For this review, use the dimensioned drawing (mm, ordinates from the lowest corner) and the shaded views. A direction names the side the tool comes from. Coordinates: 2 decimals unless noted, no trailing zeros. Loops run counter-clockwise (first coordinate to the right, second up) from the corner with the lowest first, then second, coordinate; pieces in that order, holes last. Notation, with made-up numbers: M -11,20.5 L 47,20.5 A14 cw 47,28.5 Z; hole C 29.5,78 d11. An arc over 180 degrees is marked long. One line per item, written item: value.
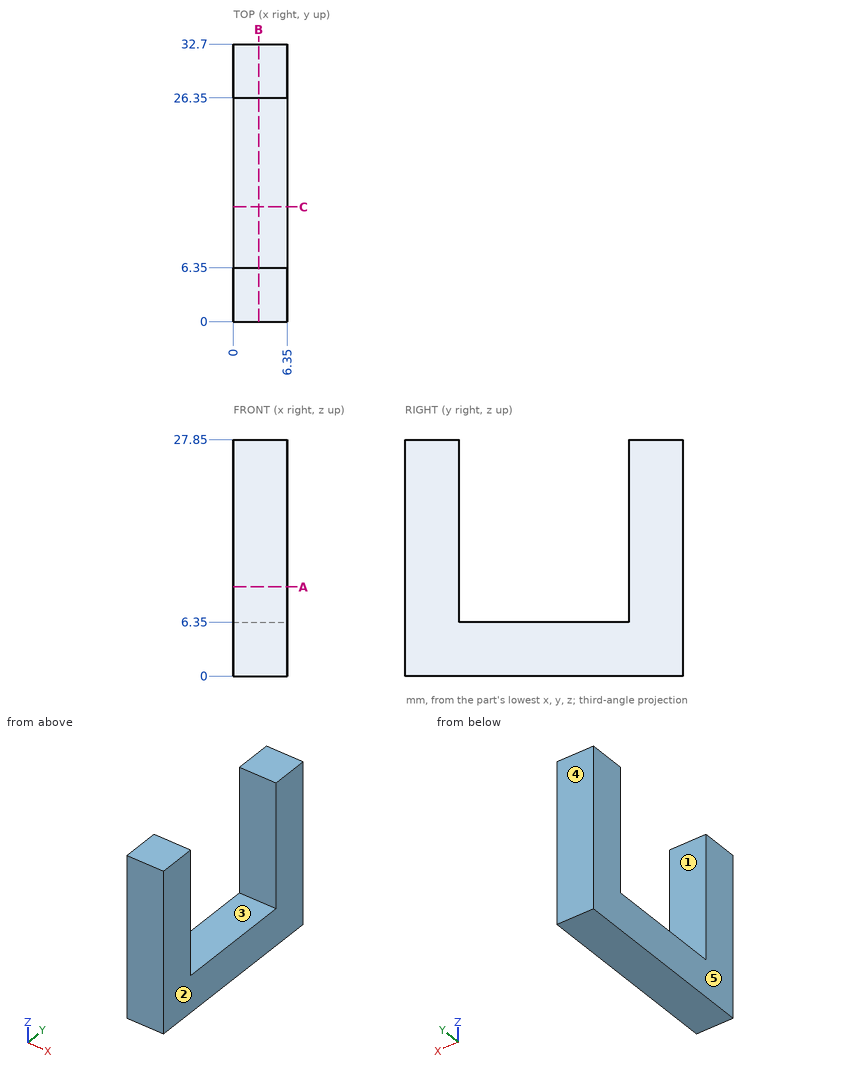
(1) We need section A-A on z = 10.5. State the section outline as (x, y) points, then the cut area to 3 significant figures.
Reply:
outline: M 0,0 L 6.35,0 L 6.35,6.35 L 0,6.35 Z; M 0,26.35 L 6.35,26.35 L 6.35,32.7 L 0,32.7 Z
area: 80.6 mm2
(2) Mouldability with a two-part tool opening along Y and no side actions: class the marked faces 3, 4 and 5 as released by +Y, released by -Y, zero draft, split by the parting line, or undercut.
Reply:
face 3: undercut
face 4: released by +Y
face 5: zero draft
(3) Tool access review of the marked faces 1 and 2: name each direction out of +Z, -Z, +X, -X, +Y, -Y from which nothing blocks a thin tool from reaching the whole face with its end or side.
Reply:
face 1: +Z, +X, -X
face 2: +Z, -Z, +X, +Y, -Y
(4) We need section C-C on y = 13.5. State the section outline as (x, z) points.
Reply:
outline: M 0,0 L 6.35,0 L 6.35,6.35 L 0,6.35 Z
(5) Insertion check: pin 1 (10 mm diameter, centred on y = 20, z = 10.5, fed in from +X); pin 2 (1.5 mm diameter, centred on x = 3.5, y = 23, fed in from +Z). Each pin has a flat end and moves straight along its axis. Give the tip position at first contact, or say it passes through.
Reply:
pin 1: stops at x = 6.35
pin 2: stops at z = 6.35
(6) We need section B-B on x = 3. State the section outline as (y, z) points, then the cut area to 3 significant figures.
Reply:
outline: M 0,0 L 32.7,0 L 32.7,27.85 L 26.35,27.85 L 26.35,6.35 L 6.35,6.35 L 6.35,27.85 L 0,27.85 Z
area: 481 mm2
(7) To check wall thickness, follow line 1 along Y through (x, z) = (5.75, 15.5); line 2 along Z through (x, y) = (2.5, 15). State the ranges of each line that lie inside material, in increasing order. Write a range as [from, to].
Reply:
line 1: y = [0, 6.35], [26.35, 32.7]
line 2: z = [0, 6.35]
